```python
from build123d import *

# Parameters (mm, degrees)
CUT_EXTRUDE1_START = -2.9464
CUT_EXTRUDE1_DEPTH = 2.9464
CUT_EXTRUDE2_DEPTH = 11.811


# Read off the part's stored shape, not the designer's step: #4-40 Tapped Hole1
with BuildPart() as part:
    # Sketch1 → Revolve1 (revolve)
    with BuildSketch(Plane(origin=(0, 0, 0), x_dir=(0, 0, -1), z_dir=(1, 0, 0)), mode=Mode.PRIVATE) as revolve1_sk:
        with BuildLine():
            Line((111.125, 0), (111.125, 2.9718))
            Line((111.125, 2.9718), (94.9452, 2.9718))
            Line((94.9452, 2.9718), (94.9452, 9.9441))
            Line((94.9452, 9.9441), (91.9988, 9.9441))
            Line((91.9988, 9.9441), (91.9988, 14.732))
            ThreePointArc((91.9988, 14.732), (91.626825612, 15.630025612), (90.7288, 16.002))
            Line((90.7288, 16.002), (56.8452, 16.002))
            Line((56.8452, 16.002), (56.8452, 16.5989))
            ThreePointArc((56.8452, 16.5989), (56.473225612, 17.496925612), (55.5752, 17.8689))
            Line((55.5752, 17.8689), (0, 17.8689))
            Line((0, 17.8689), (0, 8.0137))
            Line((0, 8.0137), (-2.286, 8.0137))
            Line((-2.286, 8.0137), (-2.286, 1.5621))
            Line((-2.286, 1.5621), (-3.5814, 1.5621))
            Line((-3.5814, 1.5621), (-3.5814, 0))
            Line((-3.5814, 0), (111.125, 0))
        make_face()
    revolve(revolve1_sk.sketch.rotate(Axis((0, 0, 3.5814), (0, 0, -1)), 90), axis=Axis((0, 0, 3.5814), (0, 0, -1)))

    # #4-40 Tapped Hole1 outline → #4-40 Tapped Hole1 (revolve, cut)
    with BuildSketch(Plane(origin=(-9, -9, 0), x_dir=(1, 0, 0), z_dir=(0, -1, 0))):
        Polygon((1.1303, -86.9188), (0, -86.239647242), (0, -91.9988), (1.1303, -91.9988), align=None)
    revolve(axis=Axis((-9, -9, 0), (0, 0, 1)), mode=Mode.SUBTRACT)

    # 4-40 Tapped Hole1 2 outline → 4-40 Tapped Hole1 2 (revolve, cut)
    with BuildSketch(Plane(origin=(9, 9, 0), x_dir=(1, 0, 0), z_dir=(0, -1, 0))):
        Polygon((1.1303, -86.9188), (0, -86.239647242), (0, -91.9988), (1.1303, -91.9988), align=None)
    revolve(axis=Axis((9, 9, 0), (0, 0, 1)), mode=Mode.SUBTRACT)

    # 4-40 Tapped Hole1 3 outline → 4-40 Tapped Hole1 3 (revolve, cut)
    with BuildSketch(Plane(origin=(9, -9, 0), x_dir=(1, 0, 0), z_dir=(0, -1, 0))):
        Polygon((1.1303, -86.9188), (0, -86.239647242), (0, -91.9988), (1.1303, -91.9988), align=None)
    revolve(axis=Axis((9, -9, 0), (0, 0, 1)), mode=Mode.SUBTRACT)

    # 4-40 Tapped Hole1 4 outline → 4-40 Tapped Hole1 4 (revolve, cut)
    with BuildSketch(Plane(origin=(-9, 9, 0), x_dir=(1, 0, 0), z_dir=(0, -1, 0))):
        Polygon((1.1303, -86.9188), (0, -86.239647242), (0, -91.9988), (1.1303, -91.9988), align=None)
    revolve(axis=Axis((-9, 9, 0), (0, 0, 1)), mode=Mode.SUBTRACT)

    # Sketch5 → Cut-Extrude1 (cut)
    with BuildSketch(Plane(origin=(0, 0, -94.9452), x_dir=(-1, 0, 0), z_dir=(0, 0, -1)).offset(CUT_EXTRUDE1_START)):
        with BuildLine():
            Line((-9.017, -4.192712226), (-9.017, 4.192712226))
            ThreePointArc((-9.017, 4.192712226), (-9.9441, 0), (-9.017, -4.192712226))
        make_face()
        with BuildLine():
            ThreePointArc((9.9441, 0), (9.709559066, 2.146995006), (9.017, 4.192712226))
            Line((9.017, 4.192712226), (9.017, -4.192712226))
            ThreePointArc((9.017, -4.192712226), (9.709559066, -2.146995006), (9.9441, 0))
        make_face()
    extrude(amount=CUT_EXTRUDE1_DEPTH, mode=Mode.SUBTRACT)

    # Sketch6 → Cut-Extrude2 (cut)
    with BuildSketch(Plane(origin=(0, 0, -111.125), x_dir=(-1, 0, 0), z_dir=(0, 0, -1))):
        Polygon((2.280914343, 68.368161202), (2.280914343, 1.905), (2.280914343, -1.905), (2.280914343, -68.368161202), (135.207236746, -68.368161202), (135.207236746, 68.368161202), align=None)
    extrude(amount=-CUT_EXTRUDE2_DEPTH, mode=Mode.SUBTRACT)


solid = part.part
```
Source: CAD feature listing. Evaluate the final solid. Frame: model axes, mm. A direction names the side the tool comes from. Coordinates: 2 decimals unless noted, no trailing zeros. Loops run counter-clockwise (first coordinate to the right, second up) from the corner with the lowest first, then second, coordinate; pieces in that order, holes last. Notation, with made-up numbers: M 70,-26.75 L 97,-26.75 A29 ccw 97,10.25 Z; hole C 32,42 d1. An arc over 180 degrees is marked long. Put each result on its own line as item: value. Start each with the question number.
1) Cut plane C-C on z = -43.5. Return the cut outline in (x, y), then the cut area to 3 significant figures.
2) Cut plane A-A on x = 0. Return the cut outline in (y, z) (3 decimals).
3) Reachability of faces 4 (the face through (-3.47, 15.62, -73.55)), 5 (the face through (4, 8, 0)), 6 (the face through (0, 0, -111.125)), 7 (the face through (0, 0, 3.581)), 8 (the face through (-2.281, 0, -105)) from +Z, -Z, +X, -X, +Y, -Y: full face, straight path, thin tool, end or side. Return the list, or none.
4) Contact query for flat-ended pins moving along their axis: pin 1 Ø1 at (x, z) = (-5.5, -58.5) entering from -Y; pin 2 Ø1 at (x, y) = (4.5, 7) entering from -Z; pin 3 Ø10 at (x, z) = (13, -28) entering from +Y. Output: stop coordinate, or through.
5) Pull-direction query (Y, two-part tool) for faces 1 (the face through (2.835, -0.893, -102.922)), 2 (the face through (0.158, -9.943, -93.451)), 3 (the face through (-9.15, 10.12, -89.42)); classes: pulls with the +Y half, pulls with the -Y half, needs draft (parallel to the pull), parting line crosses it, or undercut.
6) Cut plane B-B on z = -66.5. Return the cut outline in (x, y), then the cut area to 3 significant figures.
7) Ray query, L1, parallel to Y at x = -9, z = -87.5; L2, parallel to Z at x = -7, y = 2; L3, parallel to Z at x = -4, y = -12. Return the intervals inside material, ascending. Write a range as from..to.
The answers:
1. outline: C 0,0 d35.74
1. area: 1,000 mm²
2. outline: M -17.869,-55.575 A1.27 ccw -16.599,-56.845 L -16.002,-56.845 L -16.002,-90.729 A1.27 ccw -14.732,-91.999 L -9.944,-91.999 L -9.944,-94.945 L -2.972,-94.945 L -2.972,-111.125 L 2.972,-111.125 L 2.972,-94.945 L 9.944,-94.945 L 9.944,-91.999 L 14.732,-91.999 A1.27 ccw 16.002,-90.729 L 16.002,-56.845 L 16.599,-56.845 A1.27 ccw 17.869,-55.575 L 17.869,0 L 8.014,0 L 8.014,2.286 L 1.562,2.286 L 1.562,3.581 L -1.562,3.581 L -1.562,2.286 L -8.014,2.286 L -8.014,0 L -17.869,0 Z
3. face 4: -Z
3. face 5: +Z
3. face 6: -Z, +X, -X, +Y, -Y
3. face 7: +Z, +X, -X, +Y, -Y
3. face 8: -Z, -X, +Y, -Y
4. pin 1: stops at y = -15.2
4. pin 2: stops at z = -94.95
4. pin 3: stops at y = 15.98
5. face 1: parting line crosses it
5. face 2: pulls with the -Y half
5. face 3: undercut
6. outline: C 0,0 d32
6. area: 804 mm²
7. L1: y = -13.23..-10.13, -7.87..7.87, 10.13..13.23
7. L2: z = -94.95..2.29
7. L3: z = -92..0
